For this review, take the finished solid that the model builds, in its own axes (mm). Coordinates: 2 decimals unless noted, no trailing zeros. Loops run counter-clockwise (first coordinate to the right, second up) from the corner with the lowest first, then second, coordinate; pieces in that order, holes last. Notation, with made-up numbers: (-16.75, 84) -> (35.25, 84) arc R26 ccw to (35.25, 122) -> close; hole circle Ø8 at (-12.75, 5). An arc over 180 degrees is marked (long way). One line per item, written item: value.
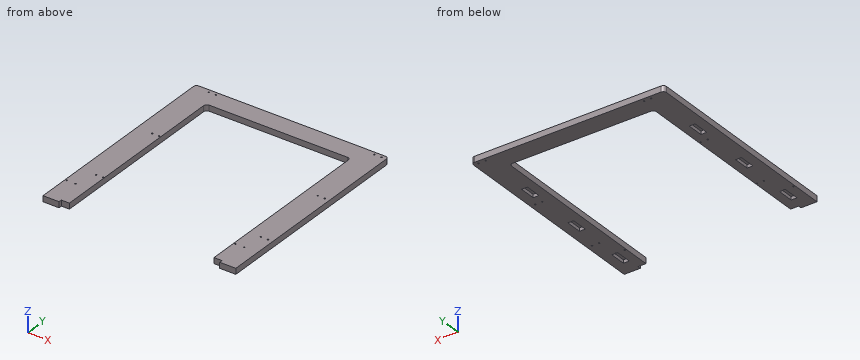
from build123d import *

# Parameters (mm, degrees)
F0_W     = 50
F0_H     = 10
F1_DEPTH = 18
F2_W     = 18
F2_H     = 50
F3_DEPTH = 10
F5_D     = 4.3
F6_R     = 10
F7_R     = 10


# Not quite as in the source:
# - a feature names something its author has since deleted; it is built from what else it names


with BuildPart() as f1:
    # F0 (on Top) → F1 (new body)
    with BuildSketch(Plane.XY):
        Polygon((600, 0), (0, 0), (0, -650), (50, -650), (75, -650), (75, -60), (525, -60), (525, -650), (550, -650), (600, -650), align=None)
        with Locations((25, -655)):
            Rectangle(F0_W, F0_H)
        with Locations((575, -655)):
            Rectangle(F0_W, F0_H)
    extrude(amount=F1_DEPTH)

    # F2 (on face) → F3 (cut)
    with BuildSketch(Plane(origin=(0, 0, 0), x_dir=(1, 0, 0), z_dir=(0, 0, -1))):
        with Locations((39, 590)):
            Rectangle(F2_W, F2_H)
        with Locations((39, 400)):
            Rectangle(F2_W, F2_H)
        with Locations((39, 200)):
            Rectangle(F2_W, F2_H)
        with Locations((561, 200)):
            Rectangle(F2_W, F2_H)
        with Locations((561, 400)):
            Rectangle(F2_W, F2_H)
        with Locations((561, 590)):
            Rectangle(F2_W, F2_H)
    extrude(amount=-F3_DEPTH, mode=Mode.SUBTRACT)

    # F5 (through all)
    with Locations(Plane.XY.offset(18)):
        with Locations((563, -10), (585, -10), (563, -255), (563, -500), (585, -500), (585, -255), (48, -10), (70, -10), (48, -255), (70, -255), (50, -500), (72, -500), (530, -565), (558, -565), (5, -565), (33, -565)):
            Hole(F5_D / 2)

    # F6
    f6_edges = [f1.edges().sort_by_distance(p)[0] for p in [
        (75, -60, 9),
        (525, -60, 9),
    ]]
    fillet(f6_edges, radius=F6_R)

    # F7
    f7_edges = [f1.edges().sort_by_distance(p)[0] for p in [
        (600, 0, 9),
        (0, 0, 9),
    ]]
    fillet(f7_edges, radius=F7_R)


solid = f1.part
1. Take a section at B-B, the plane z = 12.75. Give the number of separate pieces and of enclosed holes in the cut face, and give its area (3 significant figures).
Return value:
separate pieces: 1
enclosed holes: 16
area: 125,000 mm2
2. Take a section at D-D, the plane x = 400.5. Give the boundary of the cut face in (y, z), and give its area (3 significant figures).
Return value:
outline: (-60, 0) -> (0, 0) -> (0, 18) -> (-60, 18) -> close
area: 1,080 mm2
3. Take a section at A-A, the plane y = -391. Give the boundary of the cut face in (x, z), and give its area (3 significant figures).
Return value:
outline: (0, 0) -> (30, 0) -> (30, 10) -> (48, 10) -> (48, 0) -> (75, 0) -> (75, 18) -> (0, 18) -> close; (525, 0) -> (552, 0) -> (552, 10) -> (570, 10) -> (570, 0) -> (600, 0) -> (600, 18) -> (525, 18) -> close
area: 2,340 mm2
4. Insertion check: pin 1 Ø9 at (x, z) = (533, 11.5) entering from -Y; pin 2 Ø1.5 at (x, z) = (432, 11) entering from -Y. Each pin has a flat end and moves straight along its axis. Give the tip position at first contact, or say it passes through.
Return value:
pin 1: stops at y = -650
pin 2: stops at y = -60
5. To check wall thickness, follow probe 1 along X at (y, z) = (-565, 14.75); probe 2 along X at (y, z) = (-500, 8.5); probe 3 along Y at (x, z) = (585, 9.75). State the ranges of each line that lie inside material, in increasing order. Write a range as from..to.
Return value:
probe 1: x = 0..2.85, 7.15..30.85, 35.15..75, 525..527.85, 532.15..555.85, 560.15..600
probe 2: x = 0..47.85, 52.15..69.85, 74.15..75, 525..560.85, 565.15..582.85, 587.15..600
probe 3: y = -660..-502.15, -497.85..-257.15, -252.85..-12.15, -7.85..0
6. Take a section at C-C, the plane y = -135.5. Give the boundary of the cut face in (x, z).
Return value:
outline: (0, 0) -> (75, 0) -> (75, 18) -> (0, 18) -> close; (525, 0) -> (600, 0) -> (600, 18) -> (525, 18) -> close
